```python
from build123d import *

# Parameters (mm, degrees)
BOSS_EXTRUDE1_DEPTH = 600
FILLET1_R           = 1
SHELL3_T            = -0.2


with BuildPart() as part:
    # Sketch1 → Boss-Extrude1 (new body)
    with BuildSketch(Plane(origin=(0, 0, 0), x_dir=(1, 0, 0), z_dir=(0, 1, 0))):
        Polygon((62.497660956, -33.372417048), (51.997660956, -31.04462309), (51.997660956, -36.54462309), (57.997660956, -36.54462309), (57.997660956, -40.54462309), (51.997660956, -40.54462309), (51.997660956, -46.04462309), (62.497660956, -43.716829132), align=None)
    extrude(amount=BOSS_EXTRUDE1_DEPTH)

    # Fillet1
    fillet1_edges = [part.edges().sort_by_distance(p)[0] for p in [
        (62.497660956, 300, 43.716829132),
        (51.997660956, 300, 46.04462309),
        (51.997660956, 300, 40.54462309),
        (57.997660956, 300, 40.54462309),
        (57.997660956, 300, 36.54462309),
        (51.997660956, 300, 36.54462309),
        (51.997660956, 300, 31.04462309),
        (62.497660956, 300, 33.372417048),
    ]]
    fillet(fillet1_edges, radius=FILLET1_R)

    # Shell3
    shell3_openings = [part.faces().sort_by_distance(p)[0] for p in [
        (57.425338322, 600, 32.431348777),
        (57.425338322, 0, 32.431348777),
    ]]
    offset(amount=SHELL3_T, openings=shell3_openings, kind=Kind.INTERSECTION)


solid = part.part
```
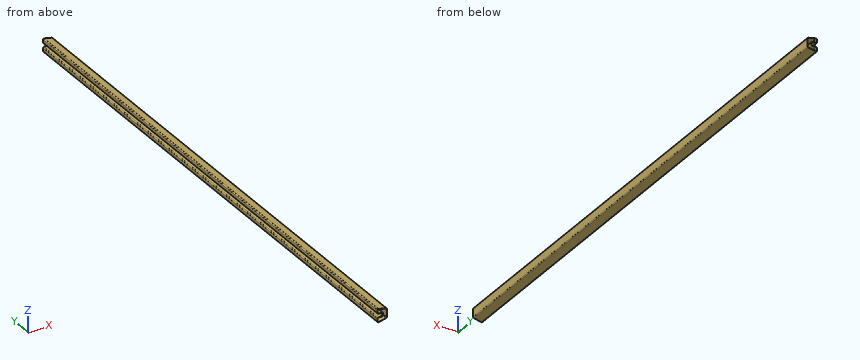
Geometry check sheet. Reference: the model listing, model coordinates, mm. Coordinates: 2 decimals unless noted, no trailing zeros. Loops run counter-clockwise (first coordinate to the right, second up) from the corner with the lowest first, then second, coordinate; pieces in that order, holes last.
Item 1: Thickness scan on line 1 (Z direction, x = 54.75, y = 525); line 2 (X direction, y = 505, z = 37.75); line 3 (X direction, y = 549, z = 43). Record the ranges inside material, lowest first.
Item 2: Go/stop test with flat-tipped pins: pin 1 Ø4.5 at (y, z) = (279, 38) entering from -X; pin 2 Ø0.6 at (y, z) = (180.5, 39) entering from -X; pin 3 Ø4 at (x, y) = (60.5, 227) entering from +Z. Record where each tip stops, or that it passes through.
Item 3: Sectioned sample at B-B, the plane x = 55. Record the boundary of the cut face in (y, z), then the cut area to 3 significant figures.
Check result:
1. line 1: z = 31.65 to 31.86, 36.34 to 36.54, 40.54 to 40.74, 45.23 to 45.43
1. line 2: x = 58 to 58.2, 62.3 to 62.5
1. line 3: x = 52 to 52.2, 62.29 to 62.49
2. pin 1: stops at x = 52.02
2. pin 2: stops at x = 58
2. pin 3: stops at z = 44.6
3. outline: (0, 31.71) - (600, 31.71) - (600, 31.92) - (0, 31.92) - close; (0, 36.34) - (600, 36.34) - (600, 36.54) - (0, 36.54) - close; (0, 40.54) - (600, 40.54) - (600, 40.74) - (0, 40.74) - close; (0, 45.17) - (600, 45.17) - (600, 45.38) - (0, 45.38) - close
3. area: 486 mm2
